Input: part model. Units: mm. Frame: model coordinates. Face numbers are marked on the shaded views. A direction names the side the tool comes from. Coordinates: 2 decimals unless noted, no trailing zeros. Loops run counter-clockwise (first coordinate to the right, second up) from the corner with the lowest first, then second, coordinate; pieces in that order, holes last.
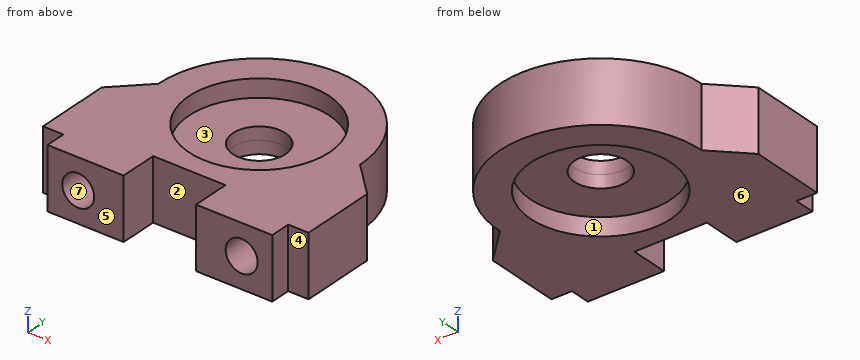
```python
from build123d import *

# Parameters (mm, degrees)
SKETCH1_R                = 8.73125
BOSS_EXTRUDE1_DEPTH      = 7.62
SKETCH3_R                = 8.7376
SKETCH3_R_2              = 3.27025
BOSS_EXTRUDE2_DEPTH      = 1.5875
BOSS_EXTRUDE2_DEPTH_BACK = 1.5875
SKETCH4_R                = 1.98374
CUT_EXTRUDE1_DEPTH       = 10.16


with BuildPart() as part:
    # Sketch1 → Boss-Extrude1 (new body)
    with BuildSketch(Plane.XY):
        with BuildLine():
            Line((4.5, 4.699), (-4.5, 4.699))
            Line((-4.5, 4.699), (-4.5, 0))
            Line((-4.5, 0), (-13.97, 0))
            Line((-13.97, 0), (-13.97, 2.54))
            Line((-13.97, 2.54), (-16.51, 2.54))
            Line((-16.51, 2.54), (-16.51, 11.90625))
            Line((-16.51, 11.90625), (-12.54125, 15.875))
            ThreePointArc((-12.54125, 15.875), (0, 28.41625), (12.54125, 15.875))
            Line((12.54125, 15.875), (16.51, 11.90625))
            Line((16.51, 11.90625), (16.51, 2.54))
            Line((16.51, 2.54), (13.97, 2.54))
            Line((13.97, 2.54), (13.97, 0))
            Line((13.97, 0), (4.5, 0))
            Line((4.5, 0), (4.5, 4.699))
        make_face()
        with Locations((0, 15.875)):
            Circle(SKETCH1_R, mode=Mode.SUBTRACT)
    extrude(amount=BOSS_EXTRUDE1_DEPTH)

    # Sketch3 → Boss-Extrude2 (add, two sides)
    with BuildSketch(Plane.XY.offset(3.81)) as boss_extrude2_sk:
        with Locations((0, 15.875)):
            Circle(SKETCH3_R)
        with Locations((0, 15.875)):
            Circle(SKETCH3_R_2, mode=Mode.SUBTRACT)
    extrude(amount=BOSS_EXTRUDE2_DEPTH)
    extrude(boss_extrude2_sk.sketch, amount=-BOSS_EXTRUDE2_DEPTH_BACK)

    # Sketch4 → Cut-Extrude1 (cut)
    with BuildSketch(Plane(origin=(0, 0, 0), x_dir=(-1, 0, 0), z_dir=(0, -1, 0))):
        with Locations((-10.16, -3.81)):
            Circle(SKETCH4_R)
        with Locations((10.16, -3.81)):
            Circle(SKETCH4_R)
    extrude(amount=-CUT_EXTRUDE1_DEPTH, mode=Mode.SUBTRACT)


solid = part.part
```
Item 1: Contact query for flat-ended pins moving along their axis: P1, Ø1.5, axis at y = 14.5, z = 2, coming from the -X side; P2, Ø3, axis at x = -5.5, z = 4, coming from the +Y side; P3, Ø8, axis at x = 4, y = 15, coming from the -Z side. Output: stop coordinate, or through.
Result:
P1: stops at x = -14.67
P2: stops at y = 27.76
P3: stops at z = 2.22
Item 2: Line query: L1, parallel to X at y = 7.5, z = 3.81; L2, parallel to Y at x = 0, z = 2.95; L3, parallel to Z at x = -10.16, y = 2.25. Output: solid intervals per line, ascending.
Result:
L1: x = -16.51 to -12.14, -8.18 to 8.18, 12.14 to 16.51
L2: y = 4.7 to 12.6, 19.15 to 28.42
L3: z = 0 to 1.83, 5.79 to 7.62
Item 3: Section query A-A (x = 0). Output: boundary loops of the cut face in (y, z).
Result:
outline: (4.7, 0) - (7.14, 0) - (7.14, 2.22) - (12.6, 2.22) - (12.6, 5.4) - (7.14, 5.4) - (7.14, 7.62) - (4.7, 7.62) - close; (19.15, 2.22) - (24.61, 2.22) - (24.61, 0) - (28.42, 0) - (28.42, 7.62) - (24.61, 7.62) - (24.61, 5.4) - (19.15, 5.4) - close
Item 4: Reachability of the marked faces 1, 2, 3 and 4 from +Z, -Z, +X, -X, +Y, -Y: full face, straight path, thin tool, end or side. Return the list, or none.
Result:
face 1: -Z
face 2: +Z, -Z, -Y
face 3: +Z
face 4: +Z, -Z, +X, -Y
Item 5: Mould query, pull axis Z, two halves, no side actions, for the marked faces 5, 6 and 7. Classes: +Z half, -Z half, draft (parallel to the pull), parting line (faces both ways), or undercut.
Result:
face 5: draft
face 6: -Z half
face 7: undercut
Item 6: Section query B-B (z = 7.25). Output: boundary loops of the cut face in (x, y) (1 decimal), then the cut area to 3 significant figures.
Result:
outline: (-16.5, 2.5) - (-14, 2.5) - (-14, 0) - (-4.5, 0) - (-4.5, 4.7) - (4.5, 4.7) - (4.5, 0) - (14, 0) - (14, 2.5) - (16.5, 2.5) - (16.5, 11.9) - (12.5, 15.9) arc R12.5 ccw to (-12.5, 15.9) - (-16.5, 11.9) - close; hole circle Ø17.5 at (0, 15.9)
area: 461 mm2
Item 7: Section query D-D (x = -10.16). Output: boundary loops of the cut face in (y, z).
Result:
outline: (0, 0) - (23.23, 0) - (23.23, 7.62) - (0, 7.62) - (0, 5.79) - (10.16, 5.79) - (10.16, 1.83) - (0, 1.83) - close
Item 8: Section query C-C (y = 23). Output: boundary loops of the cut face in (x, z), then the cut area to 3 significant figures.
Result:
outline: (-10.32, 0) - (-5.05, 0) - (-5.05, 2.22) - (5.05, 2.22) - (5.05, 0) - (10.32, 0) - (10.32, 7.62) - (5.05, 7.62) - (5.05, 5.4) - (-5.05, 5.4) - (-5.05, 7.62) - (-10.32, 7.62) - close
area: 112 mm2
